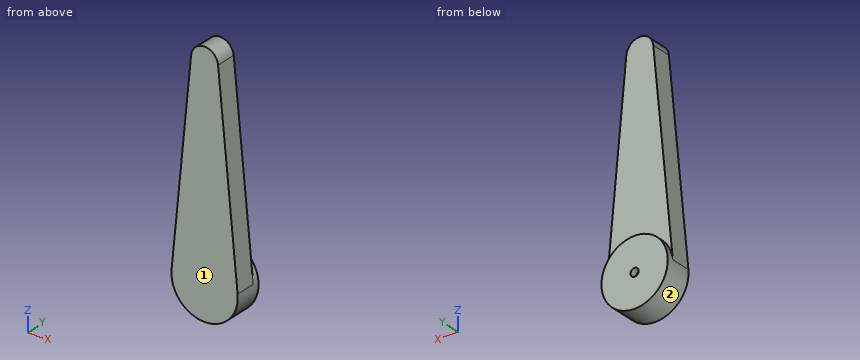
```python
from build123d import *

# Parameters (mm, degrees)
CROQUIS1_R              = 24.5
CROQUIS1_R_2            = 3
SALIENTE_EXTRUIR1_DEPTH = 20
CROQUIS3_R              = 3
SALIENTE_EXTRUIR2_DEPTH = 15


with BuildPart() as part:
    # Croquis1 → Saliente-Extruir1 (new body)
    with BuildSketch(Plane(origin=(0, 0, 0), x_dir=(1, 0, 0), z_dir=(0, 1, 0))):
        with Locations(Location((0, 0, 0), (0, 0, 270))):
            Circle(CROQUIS1_R)
        with Locations(Location((0, 0, 0), (0, 0, 270))):
            Circle(CROQUIS1_R_2, mode=Mode.SUBTRACT)
    extrude(amount=SALIENTE_EXTRUIR1_DEPTH)

    # Croquis3 → Saliente-Extruir2 (add)
    with BuildSketch(Plane.XZ):
        with BuildLine():
            Line((-9.953168117, 150.966666667), (-24.385261863, 2.368333563))
            ThreePointArc((-24.385261863, 2.368333563), (1.09e-07, 24.5), (24.385261884, 2.368333346))
            Line((24.385261884, 2.368333346), (9.953168117, 150.966666667))
            ThreePointArc((9.953168117, 150.966666667), (0, 160), (-9.953168117, 150.966666667))
        make_face()
        Circle(CROQUIS3_R)
    extrude(amount=-SALIENTE_EXTRUIR2_DEPTH)


solid = part.part
```
The model under review builds one solid part; all positions refer to its coordinate system, in mm. Face numbers are marked on the shaded views. A direction names the side the tool comes from. Round coordinates to 2 decimals unless told otherwise and drop trailing zeros. Loops run counter-clockwise (first coordinate to the right, second up) from the corner with the lowest first, then second, coordinate; pieces in that order, holes last. Notation, with made-up numbers: (8.5, 52.5) - (57.5, 52.5) arc R32 ccw to (57.5, 82.5) - close; hole circle Ø6 at (67.5, 51.25). An arc over 180 degrees is marked (long way). Use a Markdown table: item, result. Add a question column.
Q1. Add section A-A (x = 0). State the section outline as (y, z) points, plus the area to 3 significant figures.
Q2. Add section C-C (y = 17.25). State the section outline as (x, z) points.
Q3. Add section B-B (z = 0). State the section outline as (x, y) points.
Q4. For probe 1 along X at (y, z) = (16, 0); probe 2 along Y at (x, z) = (-19, 35); probe 3 along X at (y, z) = (4, 52.5), list the stretches that pass through material, from the lowest coordinate up.
Q5. Add section D-D (z = 41). State the section outline as (x, y) points.
Q6. Machinability: for the marked faces 1 and 2, which of the approach directions +Z, -Z, +X, -X, +Y, -Y give a long, thin tool a straight path to every point of the face, cutting with its end or side? Answer none if there is none.
Q7. Insertion check: pin 1 Ø3 at (x, y) = (-3.5, 4.5) entering from -Z; pin 2 Ø4 at (y, z) = (4.5, 134) entering from +X; pin 3 Ø1.5 at (y, z) = (7.5, 106) entering from -X. Each pin has a flat end and moves straight along its axis. Give the tip position at first contact, or say it passes through.
Worked answers:
| question | item | result |
|---|---|---|
| 1 | outline | (0, -24.5) - (20, -24.5) - (20, -3) - (15, -3) - (15, 3) - (20, 3) - (20, 24.5) - (15, 24.5) - (15, 160) - (0, 160) - close |
| 1 | area | 2,980 mm² |
| 2 | outline | circle Ø49 at (0, 0); hole circle Ø6 at (0, 0) |
| 3 | outline | (-24.5, 0) - (24.5, 0) - (24.5, 20) - (3, 20) - (3, 15) - (-3, 15) - (-3, 20) - (-24.5, 20) - close |
| 4 | probe 1 | -24.5 to -3, 3 to 24.5 |
| 4 | probe 2 | 0 to 15 |
| 4 | probe 3 | -19.52 to 19.52 |
| 5 | outline | (-20.63, 0) - (20.63, 0) - (20.63, 15) - (-20.63, 15) - close |
| 6 | face 1 | +Z, -Z, +X, -X, -Y |
| 6 | face 2 | +Y |
| 7 | pin 1 | z = -24.42 |
| 7 | pin 2 | x = 11.8 |
| 7 | pin 3 | x = -14.39 |
